```python
from build123d import *

# Parameters (mm, degrees)
BOSS_EXTRUDE1_DEPTH = 50
SKETCH3_R           = 2.6
CUT_EXTRUDE2_DEPTH  = 15
FILLET2_R           = 1.8
FILLET3_R           = 1.8


with BuildPart() as part:
    # Sketch1 → Boss-Extrude1 (new body, symmetric)
    with BuildSketch(Plane.XY):
        Polygon((0, 0), (50, 0), (50, 40), (23.094010768, 40), align=None)
    extrude(amount=BOSS_EXTRUDE1_DEPTH, both=True)

    # Sketch3 → Cut-Extrude2 (cut)
    with BuildSketch(Plane(origin=(0, 40, 0), x_dir=(1, 0, 0), z_dir=(0, 1, 0))):
        with Locations((35, 30)):
            Circle(SKETCH3_R)
        with Locations((35, -30)):
            Circle(SKETCH3_R)
    extrude(amount=-CUT_EXTRUDE2_DEPTH, mode=Mode.SUBTRACT)

    # Fillet2
    fillet2_edges = [part.edges().sort_by_distance(p)[0] for p in [
        (25, 0, 50),
    ]]
    fillet(fillet2_edges, radius=FILLET2_R)

    # Fillet3
    fillet3_edges = [part.edges().sort_by_distance(p)[0] for p in [
        (25, 0, -50),
    ]]
    fillet(fillet3_edges, radius=FILLET3_R)


solid = part.part
```
Part model, mm, in its own coordinate system. A direction names the side the tool comes from. Round coordinates to 2 decimals unless told otherwise and drop trailing zeros. Loops run counter-clockwise (first coordinate to the right, second up) from the corner with the lowest first, then second, coordinate; pieces in that order, holes last. Notation, with made-up numbers: (72, 28.5) -> (101, 28.5) arc R17 cw to (101, 59.5) -> close; hole circle Ø8 at (-12.5, 48). An arc over 180 degrees is marked (long way). Use one line per item in the form item = value. Start each with the question number.
Item 1: Two-plate mould, pull along X, no slides. Class faces 3 (the flat face through (35, 25, 30)), 4 (the flat face through (31, 21, 50)), 5 (the flat face through (35, 25, -30)), 6 (the flat face through (50, 20, 1)): released by +X, released by -X, zero draft, split by the parting line, or undercut.
Item 2: Tool access for faces 1 (the cylindrical face through (25.35, 0.513, 49.459)), 2 (the cylindrical face through (32.4, 32.6, 29.9)): list every direction of +Z, -Z, +X, -X, +Y, -Y with a clear straight run to the whole face (end or side of a thin tool).
Item 3: Band-saw the part on B-B (y = 29.5). List the corners of the cut face in (x, z).
Item 4: Band-saw the part on C-C (z = -30). List the corners of the cut face in (x, y), plus the area to 3 significant figures.
Item 5: Band-saw the part on D-D (z = 3). List the corners of the cut face in (x, y).
Item 6: Drop flat-ended pins along their axis: pin 1 Ø3 at (x, z) = (35, -30) entering from +Y; pin 2 Ø12 at (y, z) = (12.5, -39.5) entering from -X; pin 3 Ø8 at (x, z) = (9.5, -22.5) entering from +Y. Give the stop position or say it passes through.
Item 7: Drill centre lines: line 1 along Z through (x, y) = (35, 33); line 2 along X through (y, z) = (36, -30); line 3 along X through (y, z) = (33, -30). Where is each one in solid material? Low to high.
Item 8: Band-saw the part on A-A (x = 35). List the corners of the cut face in (y, z).
Data:
q1.face_3 = undercut
q1.face_4 = zero draft
q1.face_5 = undercut
q1.face_6 = released by +X
q2.face_1 = +Z, +X, -X, -Y
q2.face_2 = +Y
q3.outline = (17.03, -50) -> (50, -50) -> (50, 50) -> (17.03, 50) -> close; hole circle Ø5.2 at (35, -30); hole circle Ø5.2 at (35, 30)
q4.outline = (0, 0) -> (50, 0) -> (50, 40) -> (37.6, 40) -> (37.6, 25) -> (32.4, 25) -> (32.4, 40) -> (23.09, 40) -> close
q4.area = 1,460 mm^2
q5.outline = (0, 0) -> (50, 0) -> (50, 40) -> (23.09, 40) -> close
q6.pin_1 = 25
q6.pin_2 = 3.75
q6.pin_3 = 23.38
q7.line_1 = -50 to -32.6, -27.4 to 27.4, 32.6 to 50
q7.line_2 = 20.78 to 32.4, 37.6 to 50
q7.line_3 = 19.05 to 32.4, 37.6 to 50
q8.outline = (0, -48.2) arc R1.8 ccw to (1.8, -50) -> (40, -50) -> (40, -32.6) -> (25, -32.6) -> (25, -27.4) -> (40, -27.4) -> (40, 27.4) -> (25, 27.4) -> (25, 32.6) -> (40, 32.6) -> (40, 50) -> (1.8, 50) arc R1.8 ccw to (0, 48.2) -> close
